Geometry: final body of the model. Coordinates: model frame, mm. Face numbers are marked on the shaded views. A direction names the side the tool comes from. Coordinates: 2 decimals unless noted, no trailing zeros. Loops run counter-clockwise (first coordinate to the right, second up) from the corner with the lowest first, then second, coordinate; pieces in that order, holes last. Notation, with made-up numbers: M 10,24 L 29,24 A14 ccw 29,43 Z; hole C 24.5,-16.5 d10. An arc over 180 degrees is marked long. Write item = value, one per line. Start each with the question number.
```python
from build123d import *

# Parameters (mm, degrees)
SKETCH_4_W          = 60
SKETCH_4_H          = 145
EXTRUDE_1_DEPTH     = 6.5
SKETCH_5_W          = 8.25
SKETCH_5_H          = 6.5
EXTRUDE_2_DEPTH     = 2
SKETCH_7_W          = 20.8
SKETCH_7_H          = 6.5
SKETCH_7_W_2        = 20.5
EXTRUDE_3_DEPTH     = 4
EXTRUDE_START       = -60
SKETCH_7_2_W        = 20.8
SKETCH_7_2_H        = 6.5
SKETCH_7_2_W_2      = 20.5
EXTRUDE_4_DEPTH     = 2
CUT_EXTRUDE_START   = -1.8
CUT_EXTRUDE_1_DEPTH = 150.220693946
CUT_EXTRUDE_2_DEPTH = 83.004512071


with BuildPart() as part:
    # 草图4 → 凸台-拉伸1 (new body)
    with BuildSketch(Plane(origin=(0, 0, 0), x_dir=(1, 0, 0), z_dir=(0, 1, 0))):
        Rectangle(SKETCH_4_W, SKETCH_4_H)
    extrude(amount=EXTRUDE_1_DEPTH)

    # 草图5 → 凸台-拉伸2 (add)
    with BuildSketch(Plane(origin=(0, 0, -72.5), x_dir=(-1, 0, 0), z_dir=(0, 0, -1))):
        with Locations((-25.875, 3.25)):
            Rectangle(SKETCH_5_W, SKETCH_5_H)
        with Locations((-8.625, 3.25)):
            Rectangle(SKETCH_5_W, SKETCH_5_H)
        with Locations((8.625, 3.25)):
            Rectangle(SKETCH_5_W, SKETCH_5_H)
        with Locations((25.875, 3.25)):
            Rectangle(SKETCH_5_W, SKETCH_5_H)
    extrude(amount=EXTRUDE_2_DEPTH)

    # 草图7 → 凸台-拉伸3 (add)
    with BuildSketch(Plane(origin=(30, 0, 0), x_dir=(0, 0, -1), z_dir=(1, 0, 0))):
        with Locations((-62.1, 3.25)):
            Rectangle(SKETCH_7_W, SKETCH_7_H)
        with Locations((-19.983333333, 3.25)):
            Rectangle(SKETCH_7_W_2, SKETCH_7_H)
        with Locations((21.983333333, 3.25)):
            Rectangle(SKETCH_7_W_2, SKETCH_7_H)
        with Locations((64.1, 3.25)):
            Rectangle(SKETCH_7_W, SKETCH_7_H)
    extrude(amount=EXTRUDE_3_DEPTH)

    # 草图7<2> → 凸台-拉伸4 (add)
    with BuildSketch(Plane(origin=(30, 0, 0), x_dir=(0, 0, -1), z_dir=(1, 0, 0)).offset(EXTRUDE_START)):
        with Locations((-62.1, 3.25)):
            Rectangle(SKETCH_7_2_W, SKETCH_7_2_H)
        with Locations((-19.983333333, 3.25)):
            Rectangle(SKETCH_7_2_W_2, SKETCH_7_2_H)
        with Locations((21.983333333, 3.25)):
            Rectangle(SKETCH_7_2_W_2, SKETCH_7_2_H)
        with Locations((64.1, 3.25)):
            Rectangle(SKETCH_7_2_W, SKETCH_7_2_H)
    extrude(amount=-EXTRUDE_4_DEPTH)

    # 草图8 → 切除-拉伸1 (cut, through all)
    with BuildSketch(Plane.XY.offset(72.5).offset(CUT_EXTRUDE_START)):
        Polygon((10.3, 6.5), (-10.3, 6.5), (-12.5, 4.3), (-10.3, 4.3), (10.3, 4.3), (12.5, 4.3), align=None)
    extrude(amount=-CUT_EXTRUDE_1_DEPTH, mode=Mode.SUBTRACT)

    # 草图9 → 切除-拉伸2 (cut, through all)
    with BuildSketch(Plane(origin=(0, 4.3, 0), x_dir=(1, 0, 0), z_dir=(0, 1, 0))):
        Polygon((-26.875, 74.5), (-10.3, 54.5), (10.3, 54.5), (27.875, 74.5), align=None)
    extrude(amount=CUT_EXTRUDE_2_DEPTH, mode=Mode.SUBTRACT)


solid = part.part
```
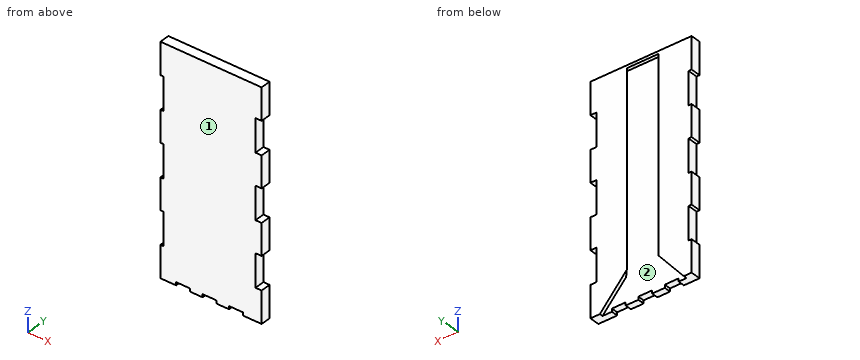
Item 1: Reachability of the marked faces 1 and 2 from +Z, -Z, +X, -X, +Y, -Y: full face, straight path, thin tool, end or side. Return the list, or none.
Item 2: Section query A-A (x = 1). Return the cut outline in (y, z), plus the area to 3 significant figures.
Item 3: Section query C-C (z = 63). Return the cut outline in (x, y), plus the area to 3 significant figures.
Item 4: Section query B-B (z = -44.5). Return the cut outline in (x, y).
Item 5: Line query: line 1 (Z direction, x = -6, y = 5); line 2 (Y direction, x = 1.5, z = 55); line 3 (X direction, y = 6, z = 33). Output: solid intervals per line, ascending. Write a range as from..to.
Item 6: First-contact query: pin 1 (2 mm diameter, centred on y = 2.5, z = 44, fed in from -X); pin 2 (1 mm diameter, centred on y = 4.5, z = -46.5, fed in from +X); pin 3 (2 mm diameter, centred on x = 15.5, y = 3, fed in from -Z). Flat tips, straight axial feed; report the tip coordinate or a pass-through.
Item 7: Section query D-D (x = 15). Return the cut outline in (y, z), plus the area to 3 significant figures.
Verdict:
q1.face_1 = +Z, -Z, +X, -X, -Y
q1.face_2 = -Z
q2.outline = M 0,-72.5 L 4.3,-72.5 L 4.3,70.7 L 6.5,70.7 L 6.5,72.5 L 0,72.5 Z
q2.area = 627 mm2
q3.outline = M -32,0 L 34,0 L 34,6.5 L 10.3,6.5 L 12.5,4.3 L -12.5,4.3 L -10.3,6.5 L -32,6.5 Z
q3.area = 379 mm2
q4.outline = M -30,0 L 30,0 L 30,6.5 L 10.3,6.5 L 12.5,4.3 L -12.5,4.3 L -10.3,6.5 L -30,6.5 Z
q5.line_1 = 70.7..72.5
q5.line_2 = 0..4.3
q5.line_3 = -30..-10.8, 10.8..30
q6.pin_1 = -30
q6.pin_2 = 30
q6.pin_3 = -72.5
q7.outline = M 0,-72.5 L 4.3,-72.5 L 4.3,-59.85 L 6.5,-59.85 L 6.5,72.5 L 0,72.5 Z
q7.area = 915 mm2
